from build123d import *

# Parameters (mm, degrees)
F1_DEPTH = 6.35
F2_W     = 3.81
F2_H     = 15.8496
F3_DEPTH = 29.21762
F4_W     = 3.04038
F4_H     = 3.81
F5_DEPTH = 51.9684
F6_W     = 1.27
F6_H     = 51.9684
F7_DEPTH = 29.21762


with BuildPart() as f1:
    # F0 (on Front) → F1 (new body)
    with BuildSketch(Plane.XZ):
        with BuildLine():
            Line((27.178, 69.088), (0, 69.088))
            Line((0, 69.088), (0, 51.9684))
            Line((0, 51.9684), (29.21762, 51.9684))
            Line((29.21762, 51.9684), (29.21762, 0))
            Line((29.21762, 0), (33.528, 0))
            Line((33.528, 0), (33.528, 62.738))
            ThreePointArc((33.528, 62.738), (31.668128, 67.228128), (27.178, 69.088))
        make_face()
    extrude(amount=F1_DEPTH)

    # F2 (on face) → F3 (cut)
    with BuildSketch(Plane(origin=(0, 0, 0), x_dir=(0, -1, 0), z_dir=(-1, 0, 0))):
        with Locations((3.175, 59.8932)):
            Rectangle(F2_W, F2_H)
    extrude(amount=-F3_DEPTH, mode=Mode.SUBTRACT)

    # F4 (on face) → F5 (cut)
    with BuildSketch(Plane(origin=(0, 0, 0), x_dir=(1, 0, 0), z_dir=(0, 0, -1))):
        with Locations((30.73781, 3.175)):
            Rectangle(F4_W, F4_H)
    extrude(amount=-F5_DEPTH, mode=Mode.SUBTRACT)

    # F6 (on face) → F7 (join, through all)
    with BuildSketch(Plane(origin=(29.21762, 0, 0), x_dir=(0, -1, 0), z_dir=(-1, 0, 0))):
        with Locations((0.635, 25.9842)):
            Rectangle(F6_W, F6_H)
    extrude(amount=F7_DEPTH)


solid = f1.part
The model under review builds one solid part; all positions refer to its coordinate system, in mm. A direction names the side the tool comes from. Round coordinates to 2 decimals unless told otherwise and drop trailing zeros. Order: outer loops, then holes, each group sorted by start corner. A loop starts at its lowest first (then second) coordinate and runs counter-clockwise, first axis right, second up. Notation, with made-up numbers: (13, 48) -> (63, 48) arc R21 cw to (63, 65) -> close; hole circle Ø9 at (50, -20). An arc over 180 degrees is marked (long way). Return JSON: item names as keys, results as strings.
1. Take a section at A-A (y = -2). Write out the cut boundary in (x, z).
Answer block:
{"outline": "(0, 67.82) -> (29.22, 67.82) -> (29.22, 51.97) -> (32.26, 51.97) -> (32.26, 0) -> (33.53, 0) -> (33.53, 62.74) arc R6.35 ccw to (27.18, 69.09) -> (0, 69.09) -> close"}
2. Insertion check: P1, Ø1, axis at x = 12, z = 19, coming from the -Y side; P2, Ø1.9, axis at x = 14, y = -3.5, coming from the -Z side; P3, Ø1.9, axis at y = -2.5, z = 59, coming from the -X side. Each pin has a flat end and moves straight along its axis. Give the tip position at first contact, or say it passes through.
Answer block:
{"P1": "stops at y = -1.27", "P2": "stops at z = 67.82", "P3": "stops at x = 29.22"}
3. Take a section at C-C (x = 11.5). Write out the cut boundary in (y, z), then the cut area to 3 significant figures.
Answer block:
{"outline": "(-6.35, 51.97) -> (-5.08, 51.97) -> (-5.08, 67.82) -> (-1.27, 67.82) -> (-1.27, 0) -> (0, 0) -> (0, 69.09) -> (-6.35, 69.09) -> close", "area": "114 mm²"}
4. The part is to be moulded in two halves that separate along Y. For faces 4 (the face through (19, -6.35, 53)), 5 (the face through (14, -5.08, 60)), 6 (the face through (17, 0, 34)), say which applies: +Y half, -Y half, draft (parallel to the pull), parting line (faces both ways), or undercut.
Answer block:
{"face 4": "-Y half", "face 5": "undercut", "face 6": "+Y half"}
5. Take a section at B-B (z = 6). Write out the cut boundary in (x, y).
Answer block:
{"outline": "(0, -1.27) -> (32.26, -1.27) -> (32.26, -5.08) -> (29.22, -5.08) -> (29.22, -6.35) -> (33.53, -6.35) -> (33.53, 0) -> (0, 0) -> close"}
6. For faces 1 (the face through (31.717, -3.131, 67.178)), 2 (the face through (29.218, -6, 26)), 3 (the face through (31, -3, 51.968)), list the 3-axis set-ups (+Z, -Z, +X, -X, +Y, -Y) from which the entire face can be reached by the end or side of a thin tool; tool diameter is ignored.
Answer block:
{"face 1": "+Z, +X, +Y, -Y", "face 2": "-Z, -X, -Y", "face 3": "-Z, -X"}
7. For L1, parallel to Y at x = 15.5, z = 49.5; L2, parallel to Y at x = 24, z = 65; L3, parallel to Z at x = 14, y = -5.25, list the stretches that pass through material, from the lowest coordinate up. Write a range as [from, to].
Answer block:
{"L1": "y = [-1.27, 0]", "L2": "y = [-6.35, -5.08], [-1.27, 0]", "L3": "z = [51.97, 69.09]"}
